Can you work these out from the model? Positions are in its coordinate system, mm. Face numbers are marked on the shaded views. A direction names the side the tool comes from. Give positions to 0.01 mm unless a question says otherwise; leave off trailing zeros. Write each loop counter-clockwise with the first axis right and the second up, starting at its lowest first coordinate (ties: lowest second). Pieces come first, ordered by that corner, then holes.
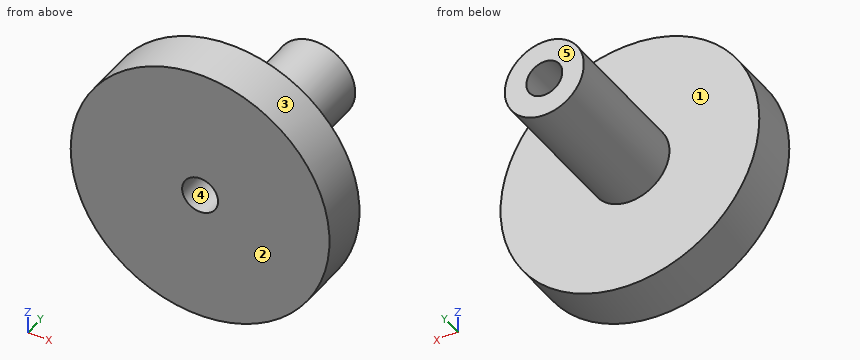
Autodesk Inventor part; units mm, degrees
ref_plane "YZ Plane" through (0, 0, 0) normal (1, 0, 0) x (0, 1, 0)
ref_plane "XZ Plane" through (0, 0, 0) normal (0, 1, 0) x (-1, 0, 0)
ref_plane "XY Plane" through (0, 0, 0) normal (0, 0, 1) x (1, 0, 0)
sketch "Sketch1" plane through (0, 0, 0) normal (0, 1, 0) x (-1, 0, 0)
  circle A0 centre (0, 0) radius 9
  dimension "d0" = 18
extrude "Extrusion1" add sketch "Sketch1" along normal blind 3.5
sketch "Sketch2" plane through (0, 3.5, 0) normal (0, 1, 0) x (1, 0, 0)
  circle A0 centre (0, 0) radius 2.75
  dimension "d3" = 5.5
extrude "Extrusion2" add sketch "Sketch2" along normal blind 10
sketch "Sketch3" plane through (0, 13.5, 0) normal (0, 1, 0) x (1, 0, 0)
  circle A0 centre (0, 0) radius 1.25
  dimension "d6" = 2.5
extrude "Extrusion3" cut sketch "Sketch3" against normal up to surface (13.5 mm away)
properties part number "Belt_Bearing_Holder"
(1) Imagine slicing it at D-D, the plane y = 7.25. Write out the boundary of the cut face in (x, z), plus the area to 3 significant figures.
Returned:
outline: circle Ø5.5 at (0, 0); hole circle Ø2.5 at (0, 0)
area: 18.8 mm2
(2) If I drill on L1, parallel to Z at x = 0, y = 7.5; L2, parallel to Y at x = 4, z = -8, over which ranges is the centre line in solid material (lowest first)?
Returned:
L1: z = -2.75 to -1.25, 1.25 to 2.75
L2: y = 0 to 3.5
(3) Imagine slicing it at B-B, the plane z = 0. Write out the boundary of the cut face in (x, y), plus the area to 4 significant figures.
Returned:
outline: (-9, 0) - (-1.25, 0) - (-1.25, 13.5) - (-2.75, 13.5) - (-2.75, 3.5) - (-9, 3.5) - close; (1.25, 0) - (9, 0) - (9, 3.5) - (2.75, 3.5) - (2.75, 13.5) - (1.25, 13.5) - close
area: 84.25 mm2
(4) Imagine slicing it at C-C, the plane y = 3.25. Write out the boundary of the cut face in (x, z).
Returned:
outline: circle Ø18 at (0, 0); hole circle Ø2.5 at (0, 0)
(5) Will these pins go through, and if not, where does the flat tip stop? P1, Ø2, axis at x = -3.5, y = 10.5, coming from the +Z side; P2, Ø1, axis at y = 3.5, z = 2, coming from the -X side.
Returned:
P1: stops at z = 1.15
P2: stops at x = -8.87
(6) Imagine slicing it at A-A, the plane x = 0. Write out the boundary of the cut face in (y, z).
Returned:
outline: (0, -9) - (3.5, -9) - (3.5, -2.75) - (13.5, -2.75) - (13.5, -1.25) - (0, -1.25) - close; (0, 1.25) - (13.5, 1.25) - (13.5, 2.75) - (3.5, 2.75) - (3.5, 9) - (0, 9) - close
(7) For the marked faces 1 and 2, which set-ups out of +Z, -Z, +X, -X, +Y, -Y let a thin tool reach every point of the face, with its end or its side?
Returned:
face 1: +Y
face 2: +Z, -Z, +X, -X, -Y
(8) If we mould it in two halves opening along Z, with no side actions, what happens to the marked faces 3, 4 and 5? For each: +Z half, -Z half, draft (parallel to the pull), parting line (faces both ways), or undercut.
Returned:
face 3: parting line
face 4: undercut
face 5: draft
